Could you check a few things on this model? Use its own coordinates, in mm. A direction names the side the tool comes from. Give positions to 0.01 mm unless a question says otherwise; leave off trailing zeros. Order: outer loops, then holes, each group sorted by start corner. A loop starts at its lowest first (then second) coordinate and runs counter-clockwise, first axis right, second up.
from build123d import *

# Parameters (mm, degrees)
CYLINDER040_R     = 3
CYLINDER040_DEPTH = 372
CYLINDER041_R     = 7
CYLINDER041_DEPTH = 3
TUBE004_R         = 40
TUBE004_R_2       = 38
TUBE004_DEPTH     = 15


with BuildPart() as pendulumshaft:
    # Cylinder040 → Cylinder040 (new body)
    with BuildSketch(Plane(origin=(0, 15, -439), x_dir=(1, 0, 0), z_dir=(0, 0, 1))):
        Circle(CYLINDER040_R)
    extrude(amount=CYLINDER040_DEPTH)


with BuildPart() as pendulumclampplate:
    # Cylinder041 → Cylinder041 (new body)
    with BuildSketch(Plane(origin=(0, 15, -70), x_dir=(1, 0, 0), z_dir=(0, 0, 1))):
        Circle(CYLINDER041_R)
    extrude(amount=CYLINDER041_DEPTH)


with BuildPart() as pendulum001:
    # Tube004 → Tube004 (new body)
    with BuildSketch(Plane(origin=(0, 22.5, -400), x_dir=(1, 0, 0), z_dir=(0, -1, 0))):
        Circle(TUBE004_R)
        Circle(TUBE004_R_2, mode=Mode.SUBTRACT)
    extrude(amount=TUBE004_DEPTH)

    # Fusion: union PendulumShaft, PendulumClampPlate
    add(pendulumshaft.part)
    add(pendulumclampplate.part)


solid = pendulum001.part
Item 1: For faces 4 (the flat face through (14.6, 22.5, -435.4)), 5 (the flat face through (1, 12, -70)), which set-ups out of +Z, -Z, +X, -X, +Y, -Y let a thin tool reach every point of the face, with its end or its side?
Findings:
face 4: +Z, -Z, +X, -X, +Y
face 5: none
Item 2: Imagine slicing it at C-C on y = 15. List the corners of the cut face in (x, z) for me, then the cut area to 3 significant figures.
Findings:
outline: (-7, -70) - (-3, -70) - (-3, -360.11) arc R40 ccw (long way) to (3, -360.11) - (3, -70) - (7, -70) - (7, -67) - (-7, -67) - close; hole (-3, -437.88) - (-3, -362.12) arc R38 ccw to start; hole (3, -437.88) arc R38 ccw to (3, -362.12) - close
area: 2,730 mm2
Item 3: Please list where these lines run through material, in increasing order: line 1 along Z through (x, y) = (0, 16.5); line 2 along Z through (x, y) = (28, 21.25); line 3 along X through (y, z) = (14, -376.5).
Findings:
line 1: z = -440 to -67
line 2: z = -428.57 to -425.69, -374.31 to -371.43
line 3: x = -32.37 to -29.86, -2.83 to 2.83, 29.86 to 32.37
Item 4: Imagine slicing it at B-B on x = 24. List the corners of the cut face in (y, z) for me.
Findings:
outline: (7.5, -432) - (22.5, -432) - (22.5, -429.46) - (7.5, -429.46) - close; (7.5, -370.54) - (22.5, -370.54) - (22.5, -368) - (7.5, -368) - close
Item 5: We'd pull the mould along Z, two halves only. Please class faces 1 (the cylindrical face through (-1.517, 8.166, -68.521)), 2 (the cylindrical face through (-4.947, 15.105, -362.323)), 3 (the flat face through (0, 15, -67)): +Z half, -Z half, draft (parallel to the pull), parting line (faces both ways), or undercut.
Findings:
face 1: draft
face 2: undercut
face 3: +Z half
Item 6: Imagine slicing it at D-D on x = -24.5. List the corners of the cut face in (y, z) for me, then the cut area to 3 significant figures.
Findings:
outline: (7.5, -431.62) - (22.5, -431.62) - (22.5, -429.05) - (7.5, -429.05) - close; (7.5, -370.95) - (22.5, -370.95) - (22.5, -368.38) - (7.5, -368.38) - close
area: 77.1 mm2
Item 7: Imagine slicing it at A-A on z = -400. List the corners of the cut face in (x, y) for me.
Findings:
outline: (-40, 7.5) - (-38, 7.5) - (-38, 22.5) - (-40, 22.5) - close; circle Ø6 at (0, 15); (38, 7.5) - (40, 7.5) - (40, 22.5) - (38, 22.5) - close
Item 8: For pin 1 (4 mm diameter, centred on x = 22.5, y = 14.5, fed in from -Z); pin 2 (5 mm diameter, centred on y = 11, z = -396.5, fed in from -X); pin 3 (5 mm diameter, centred on y = 12.5, z = -159, fed in from -X), each with a flat end and sliding along its axis, tell me the tip position at first contact or that it passes through.
Findings:
pin 1: stops at z = -434.35
pin 2: stops at x = -39.99
pin 3: stops at x = -3
